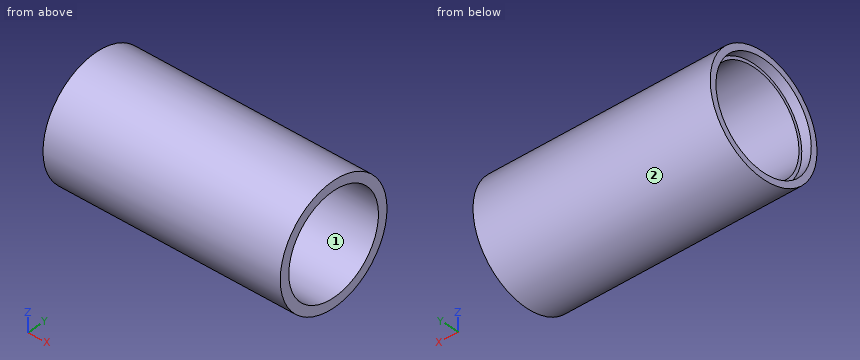
```python
from build123d import *

# Parameters (mm, degrees)
SKETCH1_R           = 9.525
BOSS_EXTRUDE1_DEPTH = 38.1
SKETCH3_R           = 8.509
CUT_EXTRUDE1_DEPTH  = 1.524
SKETCH4_R           = 8.001
CUT_EXTRUDE2_DEPTH  = 37.576


with BuildPart() as part:
    # Sketch1 → Boss-Extrude1 (new body)
    with BuildSketch(Plane(origin=(0, 0, 0), x_dir=(0, 0, -1), z_dir=(1, 0, 0))):
        Circle(SKETCH1_R)
    extrude(amount=BOSS_EXTRUDE1_DEPTH)

    # Sketch3 → Cut-Extrude1 (cut)
    with BuildSketch(Plane.ZY):
        Circle(SKETCH3_R)
    extrude(amount=-CUT_EXTRUDE1_DEPTH, mode=Mode.SUBTRACT)

    # Sketch4 → Cut-Extrude2 (cut, through all)
    with BuildSketch(Plane.ZY.offset(-1.524)):
        Circle(SKETCH4_R)
    extrude(amount=-CUT_EXTRUDE2_DEPTH, mode=Mode.SUBTRACT)


solid = part.part
```
Check sheet for the modelled part. Datum: model origin and axes. Units: mm. Face numbers are marked on the shaded views. Give positions to 0.01 mm unless a question says otherwise; leave off trailing zeros. Write each loop counter-clockwise with the first axis right and the second up, starting at its lowest first coordinate (ties: lowest second). Pieces come first, ordered by that corner, then holes.
Item 1: Cross-section at A-A (z = 0). Enter the section's corners in (x, y) (3 decimals), and give its area (3 significant figures).
Item 2: Gauge pin test, flat ends, axial feed: pin 1 (10 mm diameter, centred on x = 13, z = 3.5, fed in from -Y) (3 decimals); pin 2 (2 mm diameter, centred on x = 11, z = 6.5, fed in from -Y); pin 3 (3 mm diameter, centred on x = 31, z = -6.5, fed in from +Y); pin 4 (6 mm diameter, centred on x = 12, y = 6.5, fed in from +Z). Record the tip position at first contact, or that the pin passes through.
Item 3: Cross-section at C-C (x = 20). Enter the section's corners in (y, z) (3 decimals), and give its area (3 significant figures).
Item 4: Scan lines: L1, parallel to Y at x = 0.8, z = 0 (3 decimals); L2, parallel to Z at x = 17, y = 2; L3, parallel to Y at x = 26.5, z = 4.75. Record each from-to range of solid material in increasing order.
Item 5: Draft check along Z on the marked faces 1 and 2. Enter one of: released by +Z, released by -Z, zero draft, split by the parting line, or undercut.
Report:
1. outline: (0, -9.525) - (38.1, -9.525) - (38.1, -8.001) - (1.524, -8.001) - (1.524, -8.509) - (0, -8.509) - close; (0, 8.509) - (1.524, 8.509) - (1.524, 8.001) - (38.1, 8.001) - (38.1, 9.525) - (0, 9.525) - close
1. area: 115 mm2
2. pin 1: stops at y = -9.525
2. pin 2: stops at y = -7.78
2. pin 3: stops at y = 8.11
2. pin 4: stops at z = 8.86
3. outline: circle Ø19.05 at (0, 0); hole circle Ø16.002 at (0, 0)
3. area: 83.9 mm2
4. L1: y = -9.525 to -8.509, 8.509 to 9.525
4. L2: z = -9.31 to -7.75, 7.75 to 9.31
4. L3: y = -8.26 to -6.44, 6.44 to 8.26
5. face 1: undercut
5. face 2: split by the parting line
